Design review of the part built by this model. Coordinates are the model's own, in mm. A direction names the side the tool comes from. Coordinates: 2 decimals unless noted, no trailing zeros. Loops run counter-clockwise (first coordinate to the right, second up) from the corner with the lowest first, then second, coordinate; pieces in that order, holes last. Notation, with made-up numbers: (-1.5, 70) -> (20.5, 70) arc R22 cw to (20.5, 87) -> close; hole circle Ø8 at (82.5, 52). An arc over 180 degrees is marked (long way). Use one line per item in the form item = value. Start each with the question number.
1. Wall thickness on line 1 (X direction, y = 72, z = 0); line 2 (Z direction, x = -8.5, y = 14.5); line 3 (Y direction, x = -15.5, z = -185): over which ranges is each line inside the solid? List them lowest first. Write a range as from..to.
2. For pin 1 (5 mm diameter, centred on y = 92.5, z = -205.5, fed in from +X); pin 2 (5 mm diameter, centred on x = 13.5, y = 18.5, fed in from +Z) (3 decimals); pin 3 (12 mm diameter, centred on x = -38, y = 34.5, fed in from +Z), all flat-tipped, find the tip position at first contact; note any pin that passes through.
3. Machinability: for faces 1 (the face through (-17, 95, -225)), 2 (the face through (20, 95, -200)), 3 (the face through (-1.953, 50.7, -239.872)), 4 (the face through (-1.099, 49.3, 49.988)), which of the approach directions +Z, -Z, +X, -X, +Y, -Y give a long, thin tool a straight path to every point of the face, cutting with its end or side? Answer none if there is none.
4. Consider section D-D (x = -38). State the section outline as (y, z) points.
5. Consider section A-A (y = 14). State the section outline as (x, z) points.
6. Consider section B-B (x = 0). State the section outline as (y, z) points.
7. Consider section C-C (z = -188). State the section outline as (x, y) points, then the cut area to 3 significant figures.
8. The part is to be moulded in two halves that separate along Z. For faces 5 (the face through (-20, 95, -200)), 6 (the face through (18, 95, -225)), 7 (the face through (0, 90, -195)), say which applies: released by +Z, released by -Z, zero draft, split by the parting line, or undercut.
from build123d import *

# Parameters (mm, degrees)
SKETCH2_R           = 50
SKETCH2_R_2         = 10
BOSS_EXTRUDE1_DEPTH = 100
BOSS_EXTRUDE2_START = -100
BOSS_EXTRUDE2_DEPTH = 100
BOSS_EXTRUDE3_DEPTH = 10
BOSS_EXTRUDE4_DEPTH = 100


with BuildPart() as part:
    # Sketch2 → Boss-Extrude1 (new body)
    with BuildSketch(Plane(origin=(0, 0, 0), x_dir=(1, 0, 0), z_dir=(0, 1, 0))):
        with Locations(Location((0, 0, 0), (0, 0, 270))):
            Circle(SKETCH2_R)
        with Locations(Location((0, 0, 0), (0, 0, 270))):
            Circle(SKETCH2_R_2, mode=Mode.SUBTRACT)
    extrude(amount=BOSS_EXTRUDE1_DEPTH)

    # Sketch3 → Boss-Extrude2 (add)
    with BuildSketch(Plane(origin=(0, 100, 0), x_dir=(1, 0, 0), z_dir=(0, 1, 0)).offset(BOSS_EXTRUDE2_START)):
        with BuildLine():
            ThreePointArc((-50, 0), (0, 50), (50, 0))
            Line((50, 0), (50, 175))
            Line((50, 175), (-50, 175))
            Line((-50, 175), (-50, 0))
        make_face()
    extrude(amount=BOSS_EXTRUDE2_DEPTH)

    # Sketch4 → Boss-Extrude3 (add)
    with BuildSketch(Plane(origin=(0, 100, 0), x_dir=(1, 0, 0), z_dir=(0, 1, 0))):
        with BuildLine():
            Line((-20, 175), (20, 175))
            Line((20, 175), (20, 225))
            Line((20, 225), (15, 225))
            ThreePointArc((15, 225), (0, 210), (-15, 225))
            Line((-15, 225), (-20, 225))
            Line((-20, 225), (-20, 175))
        make_face()
    extrude(amount=-BOSS_EXTRUDE3_DEPTH)

    # Sketch4<3> → Boss-Extrude4 (add)
    with BuildSketch(Plane(origin=(0, 100, 0), x_dir=(1, 0, 0), z_dir=(0, 1, 0))):
        with BuildLine():
            ThreePointArc((-15, 225), (0, 210), (15, 225))
            Line((15, 225), (-15, 225))
        make_face()
        with BuildLine():
            Line((-15, 225), (15, 225))
            ThreePointArc((15, 225), (0, 240), (-15, 225))
        make_face()
    extrude(amount=-BOSS_EXTRUDE4_DEPTH)


solid = part.part
Geometry check:
q1.line_1 = -50..-10, 10..50
q1.line_2 = -237.36..-212.64, -175..-5.27, 5.27..49.27
q1.line_3 = 90..100
q2.pin_1 = 20
q2.pin_2 = 48.775
q2.pin_3 = 38.42
q3.face_1 = -Z, -X, +Y, -Y
q3.face_2 = -Z, +X, +Y, -Y
q3.face_3 = -Y
q3.face_4 = +Z, +Y, -Y
q4.outline = (0, -175) -> (100, -175) -> (100, 32.5) -> (0, 32.5) -> close
q5.outline = (-50, -175) -> (50, -175) -> (50, 0) arc R50 ccw to (-50, 0) -> close; circle Ø30 at (0, -225); hole circle Ø20 at (0, 0)
q6.outline = (0, -240) -> (100, -240) -> (100, -10) -> (0, -10) -> (0, -175) -> (90, -175) -> (90, -210) -> (0, -210) -> close; (0, 10) -> (100, 10) -> (100, 50) -> (0, 50) -> close
q7.outline = (-20, 90) -> (20, 90) -> (20, 100) -> (-20, 100) -> close
q7.area = 400 mm²
q8.face_5 = zero draft
q8.face_6 = released by -Z
q8.face_7 = undercut
